Build history of the part. All positions in model axes, mm. A direction names the side the tool comes from. Round coordinates to 2 decimals unless told otherwise and drop trailing zeros. Write each loop counter-clockwise with the first axis right and the second up, starting at its lowest first coordinate (ties: lowest second). Pieces come first, ordered by that corner, then holes. Notation, with made-up numbers: (18, 64) - (56, 64) arc R28 cw to (56, 87) - close; hole circle Ø1 at (2, 24.5). An arc over 180 degrees is marked (long way). Answer as a JSON object with one key per item and string values. Group by question number.
Item 1: Which spindle directions (+Z, -Z, +X, -X, +Y, -Y) get a long thin tool onto all of the face, cutting with end or side? Do faces 3 (the cylindrical face through (11.09, -0.622, 61.525)), 4 (the flat face through (9.525, 0, 100)). Say none if no direction does.
Item 2: Slice it at C-C, the plane z = 139.5. List the corners of the cut face in (x, y) (3 decimals), then the cut area to 3 significant figures.
Item 3: Probe line 1 (X direction, y = 5.5, z = 163.5) (3 decimals); line 2 (X direction, y = 10.6, z = 139.7). List the from-to ranges inside material, lowest first. Write a range as from..to.
Item 4: Slice it at A-A, the plane z = 38.1. List the corners of the cut face in (x, y) (3 decimals), then the cut area to 3 significant figures.
Item 5: Slice it at B-B, the plane x = 6.25. List the corners of the cut face in (y, z) (3 decimals), then the cut area to 3 significant figures.
Item 6: Two-plate mould, pull along Y, no slides. Class faces 1 (the cylindrical face through (-0.622, 11.09, 116.275)), 2 (the flat face through (0, -9.525, 100)): +Y half, -Y half, draft (parallel to the pull), parting line (faces both ways), or undercut.
Autodesk Inventor part; units mm, degrees
ref_plane "YZ Plane" through (0, 0, 0) normal (1, 0, 0) x (0, 1, 0)
ref_plane "XZ Plane" through (0, 0, 0) normal (0, 1, 0) x (-1, 0, 0)
ref_plane "XY Plane" through (0, 0, 0) normal (0, 0, 1) x (1, 0, 0)
sketch "Sketch1" plane through (0, 0, 0) normal (0, 0, 1) x (1, 0, 0)
  line L0 (-12.7, -12.7) -> (12.7, -12.7)
  line L1 (12.7, -12.7) -> (12.7, 12.7)
  line L2 (12.7, 12.7) -> (-12.7, 12.7)
  line L3 (-12.7, 12.7) -> (-12.7, -12.7)
  line L4 (-12.7, -12.7) -> (12.7, 12.7) construction
  line L5 (12.7, -12.7) -> (-12.7, 12.7) construction
  line L6 (9.525, -9.525) -> (-9.525, -9.525)
  line L7 (-9.525, -9.525) -> (-9.525, 9.525)
  line L8 (-9.525, 9.525) -> (9.525, 9.525)
  line L9 (9.525, 9.525) -> (9.525, -9.525)
  line L10 (9.525, -9.525) -> (-9.525, 9.525) construction
  line L11 (-9.525, -9.525) -> (9.525, 9.525) construction
  point P0 (0, 0)
  dimension "d0" = 25.4
  dimension "d1" = 25.4
  dimension "d6" = 3.175
  dimension "d7" = 3.175
extrude "Extrusion1" add sketch "Sketch1" along normal blind 203.2
sketch "Sketch6" plane through (12.7, -12.7, 0) normal (1, 0, 0) x (0, 0, -1)
  line L0 (0, 0) -> (0, 25.4)
  line L1 (0, 25.4) -> (-203.2, 25.4)
  point P0 (0, 12.7)
  point P1 (-12.7, 12.7)
  point P2 (-38.1, 12.7)
  point P3 (-63.5, 12.7)
  point P4 (-88.9, 12.7)
  point P5 (-114.3, 12.7)
  point P6 (-139.7, 12.7)
  point P7 (-165.1, 12.7)
  point P8 (-190.5, 12.7)
  dimension "d23" = 12.7
  dimension "d24" = 12.7
  dimension "d27" = 25.4
hole "Hole2" at (12.7, 0, 12.7) at (12.7, 0, 38.1) at (12.7, 0, 63.5) at (12.7, 0, 88.9) at (12.7, 0, 114.3) at (12.7, 0, 139.7) at (12.7, 0, 165.1) at (12.7, 0, 190.5) direction (-1, 0, 0) diameter 4.1402 end through all
sketch "Sketch7" plane through (-12.7, 12.7, 0) normal (0, 1, 0) x (1, 0, 0)
  line L0 (25.4, 0) -> (0, 0)
  line L1 (0, 0) -> (0, -203.2)
  point P0 (12.7, 0)
  point P1 (12.7, -12.7)
  point P2 (12.7, -38.1)
  point P3 (12.7, -63.5)
  point P4 (12.7, -88.9)
  point P5 (12.7, -114.3)
  point P6 (12.7, -139.7)
  point P7 (12.7, -165.1)
  point P8 (12.7, -190.5)
  dimension "d39" = 12.7
  dimension "d40" = 12.7
  dimension "d43" = 25.4
hole "Hole3" at (0, 12.7, 12.7) at (0, 12.7, 38.1) at (0, 12.7, 63.5) at (0, 12.7, 88.9) at (0, 12.7, 114.3) at (0, 12.7, 139.7) at (0, 12.7, 165.1) at (0, 12.7, 190.5) direction (0, -1, 0) diameter 4.1402 end through all
properties part number "C28_TK_FrontWheelGuard" material "Aluminum 6061"
Geometry says:
{
 "1": {"face 3": "+X, -X", "face 4": "+Z, -Z"},
 "2": {"outline": "(-12.7, -12.7) - (-2.06, -12.7) - (-2.06, -9.525) - (-9.525, -9.525) - (-9.525, -2.06) - (-12.7, -2.06) - close; (-12.7, 2.06) - (-9.525, 2.06) - (-9.525, 9.525) - (-2.06, 9.525) - (-2.06, 12.7) - (-12.7, 12.7) - close; (2.06, -12.7) - (12.7, -12.7) - (12.7, -2.06) - (9.525, -2.06) - (9.525, -9.525) - (2.06, -9.525) - close; (2.06, 9.525) - (9.525, 9.525) - (9.525, 2.06) - (12.7, 2.06) - (12.7, 12.7) - (2.06, 12.7) - close", "area": "230 mm^2"},
 "3": {"line 1": "x = -12.7..-9.525, 9.525..12.7", "line 2": "x = -12.7..-2.07, 2.07..12.7"},
 "4": {"outline": "(-12.7, -12.7) - (-2.07, -12.7) - (-2.07, -9.525) - (-9.525, -9.525) - (-9.525, -2.07) - (-12.7, -2.07) - close; (-12.7, 2.07) - (-9.525, 2.07) - (-9.525, 9.525) - (-2.07, 9.525) - (-2.07, 12.7) - (-12.7, 12.7) - close; (2.07, -12.7) - (12.7, -12.7) - (12.7, -2.07) - (9.525, -2.07) - (9.525, -9.525) - (2.07, -9.525) - close; (2.07, 9.525) - (9.525, 9.525) - (9.525, 2.07) - (12.7, 2.07) - (12.7, 12.7) - (2.07, 12.7) - close", "area": "230 mm^2"},
 "5": {"outline": "(-12.7, 0) - (-9.525, 0) - (-9.525, 203.2) - (-12.7, 203.2) - close; (9.525, 0) - (12.7, 0) - (12.7, 203.2) - (9.525, 203.2) - close", "area": "1,290 mm^2"},
 "6": {"face 1": "draft", "face 2": "undercut"}
}
